CAD build for the part. Positions are in the model's coordinates, mm. A direction names the side the tool comes from. Coordinates: 2 decimals unless noted, no trailing zeros. Loops run counter-clockwise (first coordinate to the right, second up) from the corner with the lowest first, then second, coordinate; pieces in that order, holes last.
1) Saw through at C-C, the plane z = 10. Write the cut outline in (x, y) (3 decimals), and give its area (3 significant figures).
2) Saw through at A-A, the plane x = 0. Write the cut outline in (y, z) (3 decimals), and give its area (3 significant figures).
3) Wall check: line 1 along Y through (x, z) = (0, 16.25) (3 decimals); line 2 along Z through (x, y) = (-0.5, -0.5); line 3 along X through (y, z) = (0.75, 14). Give the ranges that are in metal, low to high.
4) Saw through at D-D, the plane x = 2.25. Write the cut outline in (y, z).
5) Two-plate mould, pull along X, no slides. Class faces 1 (the flat face through (0, 0, -12.7)), 2 (the cylindrical face through (-1.5, 2.8, -0.3)), 3 (the flat face through (-0.7, -1.5, -19.05)): +X half, -X half, draft (parallel to the pull), parting line (faces both ways), or undercut.
6) Pin check, flat tips, straight feed: pin 1 Ø3.5 at (x, y) = (0, 0) entering from +Z; pin 2 Ø1.5 at (x, z) = (1.5, 9.5) entering from -Y; pin 3 Ø3 at (y, z) = (2, -12) entering from -X; pin 4 Ø2.5 at (x, y) = (0, 0) entering from -Z. Stop position of each tip, or through.
7) Which spindle directions (+Z, -Z, +X, -X, +Y, -Y) get a long thin tool onto all of the face, cutting with end or side? Do faces 4 (the flat face through (0, 0, 12.7)), 5 (the flat face through (-0.7, -1.5, 19.05)), 6 (the cylindrical face through (0.31, -1.39, -15.88)). Say none if no direction does.
```python
from build123d import *

# Parameters (mm, degrees)
BOSS_EXTRUDE1_START = 19.05
SKETCH13_R          = 1.4224
BOSS_EXTRUDE1_DEPTH = 6.35
CIRPATTERN1_COUNT   = 2
CIRPATTERN1_ANGLE   = 180
EXTRUDE1_DEPTH      = 19.05
EXTRUDE1_DEPTH_BACK = 19.05
SKETCH1_R           = 3.175


# Read off the part's stored shape, not the designer's step: Boss-Extrude2
with BuildPart() as part:
    # Sketch13 → Boss-Extrude1 (new body)
    with BuildSketch(Plane.XY.offset(BOSS_EXTRUDE1_START)):
        Circle(SKETCH13_R)
    extrude(amount=-BOSS_EXTRUDE1_DEPTH)

    # Boss-Extrude2 outline → Boss-Extrude2 (revolve)
    with BuildSketch(Plane.XZ):
        Polygon((1.4224, 19.05), (1.4224, 18.9738), (1.4986, 19.05), align=None)
    revolve(axis=Axis((0, 0, 0), (0, 0, 1)))


with BuildPart() as cirpattern1_1:
    # CirPattern1: pattern copy
    add(part.part.rotate(Axis((0, 3.175, 0), (0, -1, 0)), 1 * CIRPATTERN1_ANGLE / (CIRPATTERN1_COUNT - 1)))


with BuildPart() as body_3:
    # Sketch1 → Extrude1 (new, two sides: drawn at the far end of the back side and taken through both)
    with BuildSketch(Plane.XY.offset(-EXTRUDE1_DEPTH_BACK)):
        with Locations(Location((0, 0, 0), (0, 0, 180))):
            Circle(SKETCH1_R)
    extrude(amount=EXTRUDE1_DEPTH + EXTRUDE1_DEPTH_BACK)

    # Combine1: cut CirPattern1_1, part
    add(cirpattern1_1.part, mode=Mode.SUBTRACT)
    add(part.part, mode=Mode.SUBTRACT)


solid = body_3.part
```
Data:
1. outline: circle Ø6.35 at (0, 0)
1. area: 31.7 mm2
2. outline: (-3.175, -19.05) - (-1.499, -19.05) - (-1.422, -18.974) - (-1.422, -12.7) - (1.422, -12.7) - (1.422, -18.974) - (1.499, -19.05) - (3.175, -19.05) - (3.175, 19.05) - (1.499, 19.05) - (1.422, 18.974) - (1.422, 12.7) - (-1.422, 12.7) - (-1.422, 18.974) - (-1.499, 19.05) - (-3.175, 19.05) - close
2. area: 206 mm2
3. line 1: y = -3.175 to -1.422, 1.422 to 3.175
3. line 2: z = -12.7 to 12.7
3. line 3: x = -3.09 to -1.21, 1.21 to 3.09
4. outline: (-2.24, -19.05) - (2.24, -19.05) - (2.24, 19.05) - (-2.24, 19.05) - close
5. face 1: undercut
5. face 2: parting line
5. face 3: draft
6. pin 1: stops at z = 19.05
6. pin 2: stops at y = -3.09
6. pin 3: stops at x = -3.14
6. pin 4: stops at z = -12.7
7. face 4: +Z
7. face 5: +Z, +X, -X, +Y, -Y
7. face 6: -Z
